from build123d import *

# Parameters (mm, degrees)
F0_W     = 14.256329
F0_H     = 5.237018
F0_W_2   = 8.728366
F0_H_2   = 4.364182
F0_W_3   = 4.946071
F0_H_3   = 27.057927
F1_DEPTH = 4.3434


with BuildPart() as f1:
    # F0 (on Right) → F1 (new body)
    with BuildSketch(Plane.YZ):
        Polygon((22.83922, -60.81732), (22.83922, 48.578169), (9.746672, 48.578169), (9.746672, 0), (-44.369183, 0), (-44.369183, -60.81732), (-33.022311, -60.81732), (-33.022311, -14.847939), (14.110854, -14.847939), (14.110854, -60.81732), align=None)
        with Locations((-22.4028, -7.283357)):
            Rectangle(F0_W, F0_H, mode=Mode.SUBTRACT)
        with Locations((1.309254, -7.428829)):
            Rectangle(F0_W_2, F0_H_2, mode=Mode.SUBTRACT)
        with Locations((16.002, 25.448007)):
            Rectangle(F0_W_3, F0_H_3, mode=Mode.SUBTRACT)
    extrude(amount=F1_DEPTH)


solid = f1.part
Verification items for the finished model (mm, model axes). A direction names the side the tool comes from. Coordinates: 2 decimals unless noted, no trailing zeros. Loops run counter-clockwise (first coordinate to the right, second up) from the corner with the lowest first, then second, coordinate; pieces in that order, holes last. Notation, with made-up numbers: (-40, 32.25) -> (-25, 32.25) arc R10 cw to (-25, 36.25) -> close; hole circle Ø7 at (-13, 24.25). An arc over 180 degrees is marked (long way). Answer as a JSON object with one key per item and string values. Group by question number.
Item 1: Sectioned sample at B-B on z = 25.5. Record the boundary of the cut face in (x, y).
Item 2: Depth check by flat-ended pin: pin 1 (2 mm diameter, centred on x = 2.5, y = -21.5, fed in from -Z); pin 2 (1.3 mm diameter, centred on x = 1, z = 35.5, fed in from -Y); pin 3 (12 mm diameter, centred on y = 0.5, z = 18, fed in from +X). Enter the tip coordinate at first touch or a pass-through.
Item 3: Sectioned sample at D-D on y = -11.5. Record the boundary of the cut face in (x, z), plus the area to 3 significant figures.
Item 4: Scan lines: probe 1 along Y at (x, z) = (0.7, -7.5); probe 2 along Z at (x, y) = (1.6, 17.5); probe 3 along Y at (x, z) = (1.95, 35). Record each from-to range of solid material in increasing order.
Item 5: Tool access check on faces 1 (the flat face through (2, 5.673, -7)), 2 (the flat face through (2, 18, -60.817)), 3 (the flat face through (2, 14.111, -38)). Record the directions out of +Z, -Z, +X, -X, +Y, -Y that give a thin tool (end or side, any length) a straight path to the whole face; none if there is none.
Item 6: Sectioned sample at C-C on x = 1.5. Record the boundary of the cut face in (y, z).
Item 7: Sectioned sample at A-A on y = 1.5. Record the boundary of the cut face in (x, z).
Item 8: Mould release check, pull along Y, two halves, no side actions. Record for faces 4 (the flat face through (4.343, -6, -14)), 5 (the flat face through (2, 9.747, 25)), 6 (the flat face through (2, 16, 11.919)): +Y half, -Y half, draft (parallel to the pull), parting line (faces both ways), or undercut.
Evaluation:
{
 "1": {"outline": "(0, 9.75) -> (4.34, 9.75) -> (4.34, 13.53) -> (0, 13.53) -> close; (0, 18.48) -> (4.34, 18.48) -> (4.34, 22.84) -> (0, 22.84) -> close"},
 "2": {"pin 1": "stops at z = -14.85", "pin 2": "stops at y = 9.75", "pin 3": "passes through"},
 "3": {"outline": "(0, -14.85) -> (4.34, -14.85) -> (4.34, 0) -> (0, 0) -> close", "area": "64.5 mm²"},
 "4": {"probe 1": "y = -44.37 to -29.53, -15.27 to -3.05, 5.67 to 22.84", "probe 2": "z = -60.82 to 11.92, 38.98 to 48.58", "probe 3": "y = 9.75 to 13.53, 18.48 to 22.84"},
 "5": {"face 1": "+X, -X", "face 2": "-Z, +X, -X, +Y, -Y", "face 3": "-Z, +X, -X"},
 "6": {"outline": "(-44.37, -60.82) -> (-33.02, -60.82) -> (-33.02, -14.85) -> (14.11, -14.85) -> (14.11, -60.82) -> (22.84, -60.82) -> (22.84, 48.58) -> (9.75, 48.58) -> (9.75, 0) -> (-44.37, 0) -> close; hole (-29.53, -9.9) -> (-15.27, -9.9) -> (-15.27, -4.66) -> (-29.53, -4.66) -> close; hole (-3.05, -9.61) -> (5.67, -9.61) -> (5.67, -5.25) -> (-3.05, -5.25) -> close; hole (13.53, 11.92) -> (18.48, 11.92) -> (18.48, 38.98) -> (13.53, 38.98) -> close"},
 "7": {"outline": "(0, -14.85) -> (4.34, -14.85) -> (4.34, -9.61) -> (0, -9.61) -> close; (0, -5.25) -> (4.34, -5.25) -> (4.34, 0) -> (0, 0) -> close"},
 "8": {"face 4": "draft", "face 5": "-Y half", "face 6": "undercut"}
}
